Input: dimensioned drawing with shaded views. Units: mm. Origin: part minimum x, y, z. A direction names the side the tool comes from. Round coordinates to 2 decimals unless told otherwise and drop trailing zeros. Order: outer loops, then holes, each group sorted by start corner. A loop starts at its lowest first (then second) coordinate and runs counter-clockwise, first axis right, second up. Notation, with made-up numbers: (0, 34.5) - (18, 34.5) arc R19 cw to (18, 47.5) - close; hole circle Ø10 at (8.5, -1). An arc over 180 degrees is marked (long way). Put each result on its own line as item: value. Start each with the question number.
(1) Section D-D (x = 22.5). Output: boundary loops of the cut face in (y, z), and give its area (3 significant figures).
(2) Section B-B (x = 33). Output: boundary loops of the cut face in (y, z).
(3) Pin query (flat end, axial travel): P1, Ø0.9, axis at y = 49, z = 1.5, coming from the +X side; P2, Ø3.5, axis at y = 37, z = 7.5, coming from the +X side; P3, Ø3, axis at x = 9, y = 26, coming from the +Z side; P4, Ø3.5, axis at y = 92, z = 5, coming from the -X side. Return the tip coordinate at first contact, or that it passes through.
(4) Section C-C (z = 5). Output: boundary loops of the cut face in (x, y), and give its area (3 significant figures).
(5) Access query for the marked faces 1, 2 and 3. Directions: +Z, -Z, +X, -X, +Y, -Y. A direction counts if a zero-diameter tool reaches every point of the face in a straight line with its end or side. Return the directions, or none.
(6) Material intervals for L1, parallel to Y at x = 35.7, z = 5; L2, parallel to Z at x = 36, y = 92; L3, parallel to Y at x = 24.5, z = 8, sorted ascending. Write a range as [from, to].
(7) Section A-A (y = 92). Output: boundary loops of the cut face in (x, z), and give its area (3 significant figures).
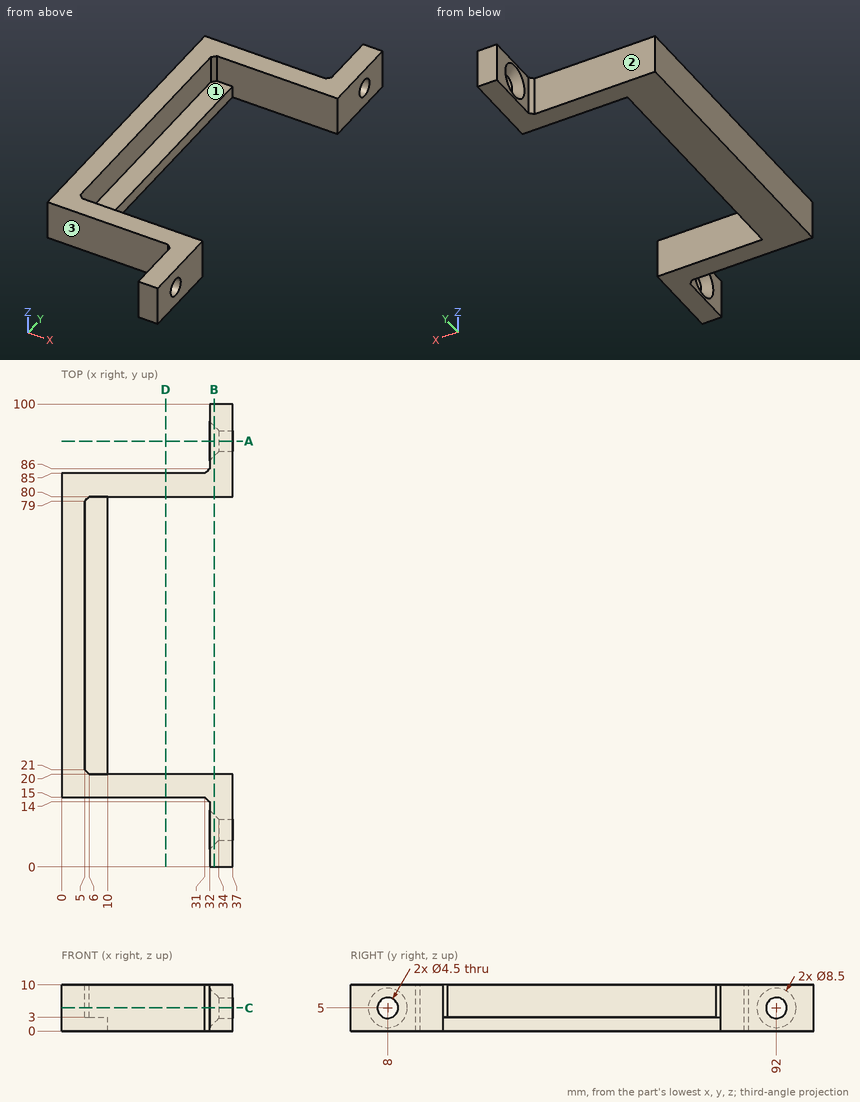
Checks:
1. outline: (15, 0) - (20, 0) - (20, 10) - (15, 10) - close; (80, 0) - (85, 0) - (85, 10) - (80, 10) - close
1. area: 100 mm²
2. outline: (0, 0) - (20, 0) - (20, 10) - (0, 10) - close; (80, 0) - (100, 0) - (100, 10) - (80, 10) - close; hole circle Ø6.5 at (8, 5); hole circle Ø6.5 at (92, 5)
3. P1: stops at x = 10
3. P2: stops at x = 5
3. P3: stops at z = 3
3. P4: passes through
4. outline: (0, 15) - (31, 15) - (32, 14) - (32, 12.25) - (34, 10.25) - (37, 10.25) - (37, 20) - (6, 20) - (5, 21) - (5, 79) - (6, 80) - (37, 80) - (37, 89.75) - (34, 89.75) - (32, 87.75) - (32, 86) - (31, 85) - (0, 85) - close; (32, 0) - (37, 0) - (37, 5.75) - (34, 5.75) - (32, 3.75) - close; (32, 96.25) - (34, 94.25) - (37, 94.25) - (37, 100) - (32, 100) - close
4. area: 769 mm²
5. face 1: +Z, +X
5. face 2: +Z, -Z, -X, +Y
5. face 3: +Z, -Z, -X, -Y
6. L1: y = [0, 5.75], [10.25, 20], [80, 89.75], [94.25, 100]
6. L2: z = [0, 2.75], [7.25, 10]
6. L3: y = [15, 20], [80, 85]
7. outline: (32, 0) - (37, 0) - (37, 2.75) - (34, 2.75) - (32, 0.75) - close; (32, 9.25) - (34, 7.25) - (37, 7.25) - (37, 10) - (32, 10) - close
7. area: 23.5 mm²
